Build history of the part. All positions in model axes, mm. A direction names the side the tool comes from. Round coordinates to 2 decimals unless told otherwise and drop trailing zeros. Write each loop counter-clockwise with the first axis right and the second up, starting at its lowest first coordinate (ties: lowest second). Pieces come first, ordered by that corner, then holes. Notation, with made-up numbers: (-13, 48.5) - (17, 48.5) arc R26 ccw to (17, 73.5) - close; hole circle Ø7 at (81, -12). An arc over 180 degrees is marked (long way). Answer as a JSON object with one key per item and string values. Group by question number.
Item 1: Probe line 1 (Y direction, x = -14.65, z = 4.65); line 2 (Y direction, x = -19, z = 3.25); line 3 (X direction, y = 32.5, z = 2.4). List the from-to ranges inside material, lowest first. Write a range as from..to.
Item 2: Two-plate mould, pull along Y, no slides. Class faces 4 (the flat face through (-19.9, 8, 3)), 5 (the flat face through (-14.25, -3.24, 2.96)), 6 (the flat face through (-18.65, 4, 3)): +Y half, -Y half, draft (parallel to the pull), parting line (faces both ways), or undercut.
Item 3: Slice it at B-B, the plane z = 1.5. List the corners of the cut face in (x, y).
Item 4: Flat gauge pins, fed straight in: pin 1 (1.5 mm diameter, centred on x = -16.5, z = 1.5, fed in from -Y); pin 2 (2.5 mm diameter, centred on x = -22.65, y = 31.341, fed in from +Z); pin 3 (1 mm diameter, centred on x = -15, z = 4, fed in from -Y); pin 4 (3 mm diameter, centred on x = -3.5, z = 4.5, fed in from +Y). Where does each tip first touch, or does it go through?
Item 5: Slice it at A-A, the plane x = -18. List the corners of the cut face in (y, z), then the cut area to 3 significant figures.
Item 6: Slice it at C-C, the plane y = 15.5. List the corners of the cut face in (x, z), then the cut area to 3 significant figures.
Item 7: Which spindle directions (+Z, -Z, +X, -X, +Y, -Y) get a long thin tool onto all of the face, cutting with end or side? Do faces 1 (the flat face through (-14.4, 8, 3)), 2 (the flat face through (-15.65, 10, 3)), 3 (the flat face through (-15, 0, 3)). Say none if no direction does.
Autodesk Inventor part; units mm, degrees
ref_plane "YZ Plane" through (0, 0, 0) normal (1, 0, 0) x (0, 1, 0)
ref_plane "XZ Plane" through (0, 0, 0) normal (0, 1, 0) x (-1, 0, 0)
ref_plane "XY Plane" through (0, 0, 0) normal (0, 0, 1) x (1, 0, 0)
sketch "Sketch1" plane through (0, 0, 0) normal (0, 0, 1) x (1, 0, 0)
  arc A0 (-22.65, 35.1889) -> (-24.65, 33.1889) centre (-22.65, 33.1889) ccw
  line L0 (-24.65, 8.5016) -> (-24.65, 33.1889)
  arc A1 (-24.65, 2.5016) -> (-24.65, 8.5016) centre (-24.65, 5.5016) ccw
  line L1 (-24.65, 0) -> (-24.65, 2.5016)
  line L2 (-18.65, 0) -> (-24.65, 0)
  line L3 (-18.65, 7) -> (-18.65, 0)
  line L4 (-19.9, 7) -> (-18.65, 7)
  line L5 (-19.9, 8.8) -> (-19.9, 7)
  line L6 (-18.65, 8.8) -> (-19.9, 8.8)
  line L7 (-18.65, 10.6) -> (-18.65, 8.8)
  line L8 (-15.65, 10.6) -> (-18.65, 10.6)
  line L9 (-15.65, 8.8) -> (-15.65, 10.6)
  line L10 (-14.4, 8.8) -> (-15.65, 8.8)
  line L11 (-14.4, 7) -> (-14.4, 8.8)
  line L12 (-15.65, 7) -> (-14.4, 7)
  line L13 (-15.65, 0) -> (-15.65, 7)
  line L14 (-14.4, 0) -> (-15.65, 0)
  line L15 (-14.1, -6.4) -> (-14.4, 0)
  line L16 (-2.3, -6.4) -> (-14.1, -6.4)
  line L17 (-2, 0) -> (-2.3, -6.4)
  line L18 (0, 0) -> (-2, 0)
  line L19 (0, 7.9) -> (0, 0)
  arc A2 (-9.6633, 32.1341) -> (0, 7.9) centre (4.112, 23.5833) ccw
  arc A3 (-9.6633, 32.1341) -> (-11.3625, 35.1889) centre (-11.3625, 33.1889) ccw
  line L20 (-22.65, 35.1889) -> (-11.3625, 35.1889)
  circle A4 centre (-14.65, 31.341) radius 1.5
  circle A5 centre (-22.65, 31.341) radius 1.5
extrude "Extrusion1" add sketch "Sketch1" along normal blind 6
properties part number "yCarWireHolder"
Geometry says:
{
 "1": {"line 1": "y = 0..7, 8.8..29.84, 32.84..35.19", "line 2": "y = 0..7, 8.8..35.19", "line 3": "x = -24.65..-23.6, -21.7..-15.6, -13.7..-9.48"},
 "2": {"face 4": "undercut", "face 5": "-Y half", "face 6": "draft"},
 "3": {"outline": "(-24.65, 0) - (-18.65, 0) - (-18.65, 7) - (-19.9, 7) - (-19.9, 8.8) - (-18.65, 8.8) - (-18.65, 10.6) - (-15.65, 10.6) - (-15.65, 8.8) - (-14.4, 8.8) - (-14.4, 7) - (-15.65, 7) - (-15.65, 0) - (-14.4, 0) - (-14.1, -6.4) - (-2.3, -6.4) - (-2, 0) - (0, 0) - (0, 7.9) arc R16.21 cw to (-9.66, 32.13) arc R2 ccw to (-11.36, 35.19) - (-22.65, 35.19) arc R2 ccw to (-24.65, 33.19) - (-24.65, 8.5) arc R3 cw to (-24.65, 2.5) - close; hole circle Ø3 at (-22.65, 31.34); hole circle Ø3 at (-14.65, 31.34)"},
 "4": {"pin 1": "stops at y = 10.6", "pin 2": "passes through", "pin 3": "stops at y = 0", "pin 4": "stops at y = 10.17"},
 "5": {"outline": "(10.6, 0) - (35.19, 0) - (35.19, 6) - (10.6, 6) - close", "area": "148 mm^2"},
 "6": {"outline": "(-24.65, 0) - (-9.94, 0) - (-9.94, 6) - (-24.65, 6) - close", "area": "88.2 mm^2"},
 "7": {"face 1": "+Z, -Z", "face 2": "+Z, -Z, -Y", "face 3": "+Z, -Z, -X, -Y"}
}
